from build123d import *

# Parameters (mm, degrees)
EXTRUDE_1_DEPTH     = 3
FILLET_1_R          = 40
SKETCH_2_R          = 5
CUT_EXTRUDE_1_DEPTH = 5
SKETCH_3_R          = 5
CUT_EXTRUDE_2_DEPTH = 5


with BuildPart() as part:
    # 草图1 → 凸台-拉伸1 (new body)
    with BuildSketch(Plane(origin=(0, 0, 0), x_dir=(1, 0, 0), z_dir=(0, 1, 0))):
        with BuildLine():
            Line((-23.136391963, 12.14008034), (-4.550043431, 6.580053554))
            ThreePointArc((-4.550043431, 6.580053554), (7.664409986, -2.292775515), (-7.416012825, -3.000458929))
            Line((-7.416012825, -3.000458929), (-19.543612326, 0.627460668))
            Line((-19.543612326, 0.627460668), (-82.193752502, -77.622539332))
            ThreePointArc((-82.193752502, -77.622539332), (-95, -85.61753733), (-90, -71.372539332))
            Line((-90, -71.372539332), (-23.136391963, 12.14008034))
        make_face()
    extrude(amount=EXTRUDE_1_DEPTH)

    # 圆角1
    # the kernel refuses this fillet: 40 mm, written as the material it adds along each edge
    with BuildSketch(Plane(origin=(-19.543612326, 0, -0.627460668), x_dir=(0.9580512482944434, 0, 0.2865969393441921), z_dir=(0, 1, 0))) as fillet_1_piece_1:
        with BuildLine():
            CenterArc((28.245446023, -36.838167986), FILLET_1_R, 112.934019548, 45.038121995)
            Line((-8.834618101, -21.835873341), (-9.576219383, -21.535827448))
            Line((-9.576219383, -21.535827448), (-0.741601282, 0.300045893))
            Line((-0.741601282, 0.300045893), (0, 0.8))
            ThreePointArc((0, 0.8), (6.329306247, 0.8), (12.346875823, 0.73676336))
            Line((12.346875823, 0.73676336), (12.658612494, 0))
        make_face()
    extrude(amount=3)
    # the kernel refuses this fillet: 40 mm, written as the material it takes off along each edge
    with BuildSketch(Plane(origin=(-23.136391963, -65.299644029, -12.14008034), x_dir=(0.9580512482944434, 0, 0.2865969393441925), z_dir=(0, 1, 0))) as fillet_1_2_piece_1:
        with BuildLine():
            CenterArc((27.283619124, -39.215444523), FILLET_1_R, 101.366634115, 56.605507428)
            Line((-9.796444999, -24.213149878), (-10.538046282, -23.913103985))
            Line((-10.538046282, -23.913103985), (-0.741601282, 0.300045893))
            Line((-0.741601282, 0.300045893), (0, 0.8))
            ThreePointArc((0, 0.8), (9.700080536, 0.8), (19.24249191, 0.78430889))
            Line((19.24249191, 0.78430889), (19.400161071, 0))
        make_face()
    extrude(amount=133.599288058, mode=Mode.SUBTRACT)

    # 草图2 → 切除-拉伸1 (cut)
    with BuildSketch(Plane(origin=(0, 3, 0), x_dir=(1, 0, 0), z_dir=(0, 1, 0))):
        with Locations(Location((-90, -79.372539332, 0), (0, 0, 270))):
            Circle(SKETCH_2_R)
    extrude(amount=-CUT_EXTRUDE_1_DEPTH, mode=Mode.SUBTRACT)

    # 草图3 → 切除-拉伸2 (cut)
    with BuildSketch(Plane(origin=(0, 3, 0), x_dir=(1, 0, 0), z_dir=(0, 1, 0))):
        with Locations(Location((0, 0, 0), (0, 0, 270))):
            Circle(SKETCH_3_R)
    extrude(amount=-CUT_EXTRUDE_2_DEPTH, mode=Mode.SUBTRACT)


solid = part.part
Geometry: final body of the model. Coordinates: model frame, mm. A direction names the side the tool comes from. Give positions to 0.01 mm unless a question says otherwise; leave off trailing zeros. Loops run counter-clockwise (first coordinate to the right, second up) from the corner with the lowest first, then second, coordinate; pieces in that order, holes last. Notation, with made-up numbers: (-26.5, 12.5) -> (-11.5, 12.5) arc R37 cw to (-11.5, 49.5) -> close; hole circle Ø4 at (66, 25.5). An arc over 180 degrees is marked (long way). Put each result on its own line as item: value.
1. Cut plane B-B (y = 1.25). Return the cut outline in (x, z), plus the area to 3 significant figures.
Taken from the geometry:
outline: (-90, 71.37) -> (-39.46, 8.25) arc R40 ccw to (-4.55, -6.58) arc R8 ccw (long way) to (-7.42, 3) arc R40 cw to (-34.27, 17.76) -> (-82.19, 77.62) arc R8 ccw (long way) to start; hole circle Ø10 at (-90, 79.37); hole circle Ø10 at (0, 0)
area: 1,380 mm2
2. Cut plane C-C (z = 0). Return the cut outline in (x, y), plus the area to 3 significant figures.
Taken from the geometry:
outline: (-30.47, 0) -> (-5, 0) -> (-5, 3) -> (-30.47, 3) -> close; (5, 0) -> (8, 0) -> (8, 3) -> (5, 3) -> close
area: 85.4 mm2
3. Ray query, line 1 along X through (y, z) = (2.3, 0); line 2 along Z through (x, y) = (-88, 1.8); line 3 along Z through (x, y) = (-88.5, 1.85). Return the intervals inside material, ascending. Write a range as [from, to].
Taken from the geometry:
line 1: x = [-30.47, -5], [5, 8]
line 2: z = [68.87, 74.79], [83.96, 87.12]
line 3: z = [69.5, 74.6], [84.14, 87.23]
4. Cut plane A-A (x = 0). Return the cut outline in (y, z).
Taken from the geometry:
outline: (0, -8) -> (3, -8) -> (3, -5) -> (0, -5) -> close; (0, 5) -> (3, 5) -> (3, 8) -> (0, 8) -> close
5. Pull-direction query (X, two-part tool) for faces 1 (the flat face through (-48, 0, 29)), 2 (the flat face through (-57.89, 1.48, 47.27)), 3 (the cylindrical face through (-4.88, 1.52, -1.08)); classes: released by +X, released by -X, zero draft, split by the parting line, or undercut.
Taken from the geometry:
face 1: zero draft
face 2: released by +X
face 3: undercut
6. Pin query (flat end, axial travel): P1, Ø8, axis at x = -90, z = 79.37, coming from the +Y side. Return the tip coordinate at first contact, or that it passes through.
Taken from the geometry:
P1: passes through
7. Cut plane D-D (z = 13). Return the cut outline in (x, y), plus the area to 3 significant figures.
Taken from the geometry:
outline: (-43.26, 0) -> (-29.77, 0) -> (-29.77, 3) -> (-43.26, 3) -> close
area: 40.5 mm2
8. Set-up query: faces 4 (the cylindrical face through (-22.117, 1.479, 7.602)), 5 (the flat face through (-48, 3, 29)). Return all of +Z, -Z, +X, -X, +Y, -Y with unobstructed straight access to the full face (end or side cutting, diameter ignored); none if empty.
Taken from the geometry:
face 4: +Z, +Y, -Y
face 5: +Z, -Z, +X, -X, +Y
